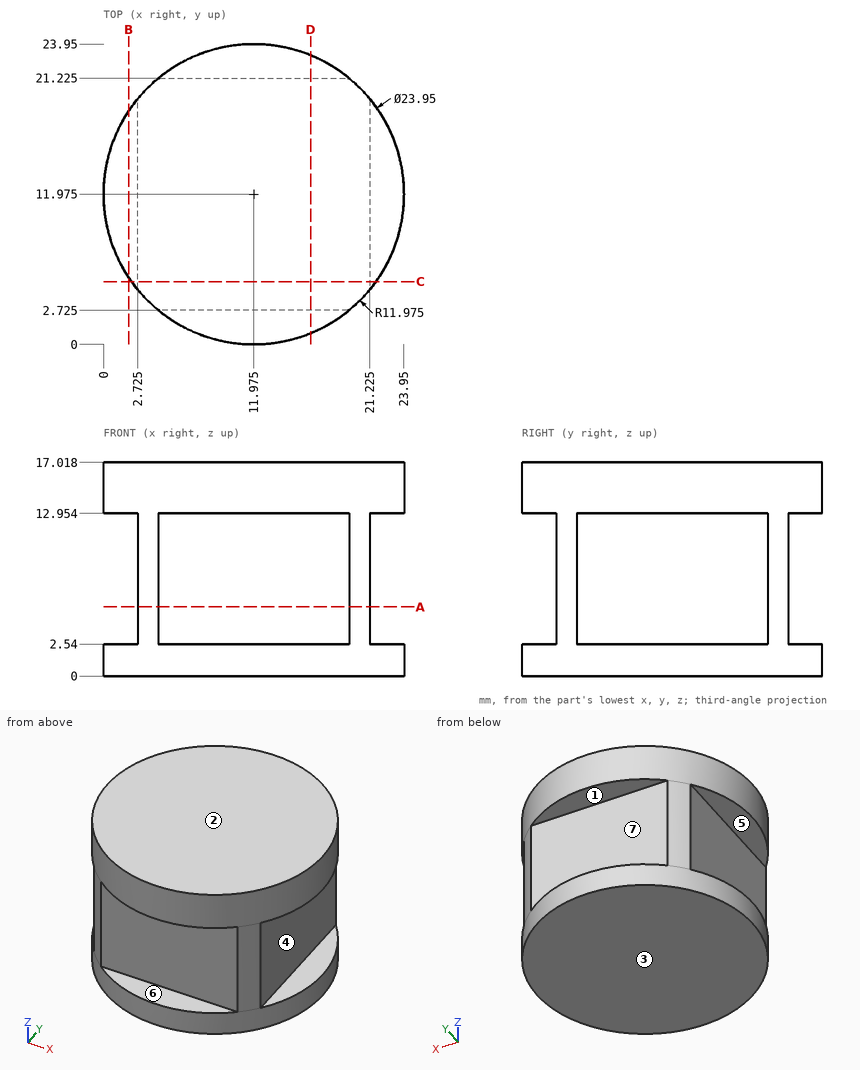
Geometry: see drawing. Coordinates: mm, zero at the bounding-box minimum. A direction names the side the tool comes from. Coordinates: 2 decimals unless noted, no trailing zeros. Order: outer loops, then holes, each group sorted by start corner. A loop starts at its lowest first (then second) coordinate and runs counter-clockwise, first axis right, second up. Notation, with made-up numbers: (68.5, -14) -> (122.5, -14) arc R9 cw to (122.5, 0) -> close; hole circle Ø10 at (43.25, 7.25). An arc over 180 degrees is marked (long way). Write each question's results on one line, items separated by ' | '. Start each with the question number.
1) Cut plane A-A, the plane z = 5.5. Output: boundary loops of the cut face in (x, y) (3 decimals).
2) Set-up query: the marked faces 4, 5, 6 and 7. Return all of +Z, -Z, +X, -X, +Y, -Y with unobstructed straight access to the full face (end or side cutting, diameter ignored); none if empty.
3) First-contact query: pin 1 (0.8 mm diameter, centred on x = 22.5, y = 11, fed in from -Z); pin 2 (2 mm diameter, centred on x = 5.5, z = 2.5, fed in from +Y); pin 3 (5 mm diameter, centred on x = 15, z = 7, fed in from -Y) (3 decimals); pin 4 (5 mm diameter, centred on y = 15.5, z = 9.5, fed in from -X) (3 decimals). Flat tips, straight axial feed; report the tip coordinate or a pass-through.
4) Cut plane D-D, the plane x = 16.5. Output: boundary loops of the cut face in (y, z) (3 decimals), and give its area (3 significant figures).
5) Cut plane B-B, the plane x = 2. Output: boundary loops of the cut face in (y, z).
6) Material intervals for line 1 along Y through (x, z) = (8, 11.75) (3 decimals); line 2 along Z through (x, y) = (23, 9), sorted ascending.
7) Mould query, pull axis Z, two halves, no side actions, for the marked faces 1, 2 and 3. Classes: released by +Z, released by -Z, zero draft, split by the parting line, or undercut.
8) Cut plane C-C, the plane y = 5. Output: boundary loops of the cut face in (x, z) (3 decimals), and give its area (3 significant figures).
Checks:
1) outline: (2.725, 4.37) arc R11.975 ccw to (4.37, 2.725) -> (19.58, 2.725) arc R11.975 ccw to (21.225, 4.37) -> (21.225, 19.58) arc R11.975 ccw to (19.58, 21.225) -> (4.37, 21.225) arc R11.975 ccw to (2.725, 19.58) -> close
2) face 4: +X, +Y, -Y | face 5: -X, +Y, -Y | face 6: +X, -X, -Y | face 7: +X, -X, +Y
3) pin 1: z = 0 | pin 2: y = 22.63 | pin 3: y = 2.725 | pin 4: x = 2.725
4) outline: (0.888, 0) -> (23.062, 0) -> (23.062, 2.54) -> (21.225, 2.54) -> (21.225, 12.954) -> (23.062, 12.954) -> (23.062, 17.018) -> (0.888, 17.018) -> (0.888, 12.954) -> (2.725, 12.954) -> (2.725, 2.54) -> (0.888, 2.54) -> close | area: 339 mm^2
5) outline: (5.35, 0) -> (18.6, 0) -> (18.6, 2.54) -> (5.35, 2.54) -> close; (5.35, 12.95) -> (18.6, 12.95) -> (18.6, 17.02) -> (5.35, 17.02) -> close
6) line 1: 2.725 to 21.225 | line 2: 0 to 2.54, 12.95 to 17.02
7) face 1: undercut | face 2: released by +Z | face 3: released by -Z
8) outline: (2.241, 0) -> (21.709, 0) -> (21.709, 2.54) -> (21.225, 2.54) -> (21.225, 12.954) -> (21.709, 12.954) -> (21.709, 17.018) -> (2.241, 17.018) -> (2.241, 12.954) -> (2.725, 12.954) -> (2.725, 2.54) -> (2.241, 2.54) -> close | area: 321 mm^2
